Answer from the drawing. Dimensions are ordinates in mm from the lowest x, y and z of the part. A direction names the side the tool comes from. Coordinates: 2 decimals unless noted, no trailing zeros. Write each loop counter-clockwise with the first axis right and the second up, starting at its lowest first coordinate (ties: lowest second). Pieces come first, ordered by that corner, then holes.
(1) The part is cut by section C-C on y = 1.25. Determine the outline of the cut face in (x, z), plus the area to 3 significant figures.
(2) Which of the six approach directions +Z, -Z, +X, -X, +Y, -Y give full straight-line access (tool end or side, diameter ignored) to the marked faces 1 and 2?
(3) The part is cut by section B-B on z = 15. Determine the outline of the cut face in (x, y), plus the area to 3 significant figures.
(4) Given P1, Ø10, axis at y = 4, z = 4, coming from the -X side; P2, Ø9, axis at x = 15, z = 15, coming from the -Y side; P3, Ø1.8, axis at y = 16, z = 7.5, coming from the +X side, each flat-ended and moving along its own axis, determine where each tip first touches the part or whether it passes through.
(5) Straight lines are drawn through the part: line 1 (Z direction, x = 15, y = 3.5); line 2 (Y direction, x = 28.95, z = 7.5); line 3 (Y direction, x = 12.25, z = 15.5). For each, find the intervals that lie inside material, in ascending order.
(6) The part is cut by section A-A on y = 16. Determine the outline of the cut face in (x, z).
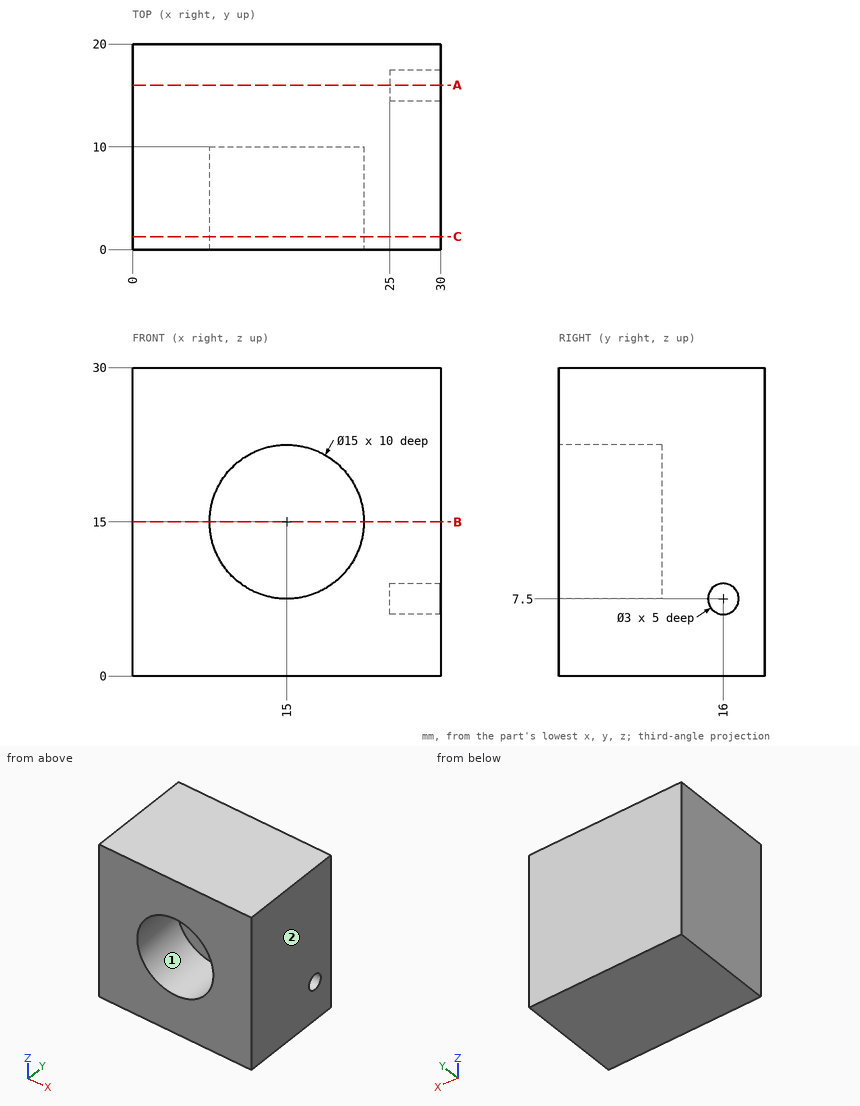
Model answer:
1. outline: (0, 0) - (30, 0) - (30, 30) - (0, 30) - close; hole circle Ø15 at (15, 15)
1. area: 723 mm2
2. face 1: -Y
2. face 2: +Z, -Z, +X, +Y, -Y
3. outline: (0, 0) - (7.5, 0) - (7.5, 10) - (22.5, 10) - (22.5, 0) - (30, 0) - (30, 20) - (0, 20) - close
3. area: 450 mm2
4. P1: stops at x = 0
4. P2: stops at y = 10
4. P3: stops at x = 25
5. line 1: z = 0 to 7.5, 22.5 to 30
5. line 2: y = 0 to 14.5, 17.5 to 20
5. line 3: y = 10 to 20
6. outline: (0, 0) - (30, 0) - (30, 6) - (25, 6) - (25, 9) - (30, 9) - (30, 30) - (0, 30) - close
